from build123d import *

# Parameters (mm, degrees)
SKETCH1_R           = 32.5
BOSS_EXTRUDE1_DEPTH = 34.793
SKETCH4_W           = 66.380152204
SKETCH4_H           = 3
CUT_EXTRUDE1_DEPTH  = 5
SKETCH5_R           = 8
SKETCH5_R_2         = 6
CUT_EXTRUDE2_DEPTH  = 2


with BuildPart() as part:
    # Sketch1 → Boss-Extrude1 (new body)
    with BuildSketch(Plane(origin=(0, 0, 0), x_dir=(1, 0, 0), z_dir=(0, 1, 0))):
        Circle(SKETCH1_R)
    extrude(amount=BOSS_EXTRUDE1_DEPTH)

    # Sketch4 → Cut-Extrude1 (cut)
    with BuildSketch(Plane(origin=(0, 34.793, 0), x_dir=(1, 0, 0), z_dir=(0, 1, 0))):
        Rectangle(SKETCH4_W, SKETCH4_H)
    extrude(amount=-CUT_EXTRUDE1_DEPTH, mode=Mode.SUBTRACT)

    # Sketch5 → Cut-Extrude2 (cut)
    with BuildSketch(Plane.XZ):
        Circle(SKETCH5_R)
        Circle(SKETCH5_R_2, mode=Mode.SUBTRACT)
    extrude(amount=-CUT_EXTRUDE2_DEPTH, mode=Mode.SUBTRACT)


solid = part.part
For this review, take the finished solid that the model builds, in its own axes (mm). A direction names the side the tool comes from. Give positions to 0.01 mm unless a question says otherwise; leave off trailing zeros. Loops run counter-clockwise (first coordinate to the right, second up) from the corner with the lowest first, then second, coordinate; pieces in that order, holes last. Notation, with made-up numbers: M -19.5,23 L 33.5,23 A20 ccw 33.5,28 Z; hole C 73.25,81.5 d11. An arc over 180 degrees is marked long. Answer as a JSON object with one key per item and string values. Group by question number.
Q1. Add section A-A on z = 0. Give the boundary of the cut face in (x, y).
Q2. Insertion check: P1, Ø1.5, axis at x = -2, y = 32, coming from the -Z side; P2, Ø1.5, axis at x = 5, y = 32.5, coming from the +Z side; P3, Ø3, axis at y = 7, z = -24, coming from the +X side. Each pin has a flat end and moves straight along its axis. Give the tip position at first contact, or say it passes through.
Q3. Add section C-C on y = 24. Give the boundary of the cut face in (x, z), and give its area (3 significant figures).
Q4. For probe 1 along Z at (x, y) = (0, 1.15); probe 2 along Z at (x, y) = (-1.5, 24); probe 3 along Z at (x, y) = (29, 19), list the stretches that pass through material, from the lowest coordinate up. Write a range as [from, to].
Q5. Tool access review of faces 4 (the flat face through (7, 0, 7)), 5 (the cylindrical face through (-1.73, 0.99, -7.81)), 6 (the flat face through (0, 29.793, 0)): name each direction out of +Z, -Z, +X, -X, +Y, -Y from which nothing blocks a thin tool from reaching the whole face with its end or side.
Q6. Add section B-B on x = 26. Give the boundary of the cut face in (y, z), and give its area (3 significant figures).
Q7. Add section D-D on x = 17.5. Give the boundary of the cut face in (y, z).
Q8. Mouldability with a two-part tool opening along Z and no side actions: class faces 1 (the cylindrical face through (-6, 1, 0)), 2 (the flat face through (0, 34.793, 13)), 3 (the cylindrical face through (31, 17.15, -9.76)) as +Z half, -Z half, draft (parallel to the pull), parting line (faces both ways), or undercut.
Checked values:
{
 "1": {"outline": "M -32.5,0 L -8,0 L -8,2 L -6,2 L -6,0 L 6,0 L 6,2 L 8,2 L 8,0 L 32.5,0 L 32.5,29.79 L -32.5,29.79 Z"},
 "2": {"P1": "z = -32.48", "P2": "z = 32.22", "P3": "x = 23.45"},
 "3": {"outline": "C 0,0 d65", "area": "3,320 mm²"},
 "4": {"probe 1": "[-32.5, -8], [-6, 6], [8, 32.5]", "probe 2": "[-32.47, 32.47]", "probe 3": "[-14.67, 14.67]"},
 "5": {"face 4": "+Z, -Z, +X, -X, -Y", "face 5": "-Y", "face 6": "+X, -X, +Y"},
 "6": {"outline": "M 0,-19.5 L 34.79,-19.5 L 34.79,-1.5 L 29.79,-1.5 L 29.79,1.5 L 34.79,1.5 L 34.79,19.5 L 0,19.5 Z", "area": "1,340 mm²"},
 "7": {"outline": "M 0,-27.39 L 34.79,-27.39 L 34.79,-1.5 L 29.79,-1.5 L 29.79,1.5 L 34.79,1.5 L 34.79,27.39 L 0,27.39 Z"},
 "8": {"face 1": "undercut", "face 2": "draft", "face 3": "parting line"}
}
